CAD build for the part. Positions are in the model's coordinates, mm. A direction names the side the tool comes from. Coordinates: 2 decimals unless noted, no trailing zeros. Order: outer loops, then holes, each group sorted by start corner. A loop starts at its lowest first (then second) coordinate and runs counter-clockwise, first axis right, second up.
from build123d import *

# Parameters (mm, degrees)
PAD_DEPTH     = 2.5
SKETCH002_W   = 6.25
SKETCH002_H   = 30
SKETCH002_W_2 = 10
SKETCH002_H_2 = 35
POCKET_DEPTH  = 1.5


with BuildPart() as part:
    # Sketch → Pad (new body)
    with BuildSketch(Plane.XY):
        Polygon((-10, 14.125), (5, 14.125), (12.25, 7.5), (102.25, 7.5), (102.25, -7.5), (12.25, -7.5), (5, -14.125), (-10, -14.125), (-10, -9.125), (0, -9.125), (0, 9.125), (-10, 9.125), align=None)
    extrude(amount=PAD_DEPTH)

    # Sketch002 → Pocket (cut)
    with BuildSketch(Plane.XY.offset(2.5)):
        with Locations((94.125, 0)):
            Rectangle(SKETCH002_W, SKETCH002_H)
        with Locations((-7, 0)):
            Rectangle(SKETCH002_W_2, SKETCH002_H_2)
    extrude(amount=-POCKET_DEPTH, mode=Mode.SUBTRACT)


solid = part.part
1) Which spindle directions (+Z, -Z, +X, -X, +Y, -Y) get a long thin tool onto all of the face, cutting with end or side? Do faces 4 (the flat face through (57, 7.5, 1)), 5 (the flat face through (58, -7.5, 1)), 6 (the flat face through (-3.8, 9.125, 0.7)), 7 (the flat face through (-6, -12, 1)). Say none if no direction does.
2) Slice it at B-B (y = 4.75). List the corners of the cut face in (x, z), plus the area to 3 significant figures.
3) Drill centre lines: probe 1 along X at (y, z) = (0, 2); probe 2 along Y at (x, z) = (76, 1.2); probe 3 along X at (y, z) = (-1.5, 0.15). Where is each one in solid material? Low to high.
4) Slice it at A-A (z = 1.75). List the corners of the cut face in (x, y) (3 decimals), plus the area to 3 significant figures.
5) Slice it at C-C (x = 79.5). List the corners of the cut face in (y, z).
6) Slice it at D-D (y = -10.5). List the corners of the cut face in (x, z), plus the area to 3 significant figures.
7) Two-plate mould, pull along Y, no slides. Class faces 1 (the flat face through (-6, 12, 1)), 2 (the flat face through (-1, -14.125, 1)), 3 (the flat face through (0, 0, 1)): released by +Y, released by -Y, zero draft, split by the parting line, or undercut.
8) Pin check, flat tips, straight feed: P1, Ø1.5, axis at x = 26, z = 1.5, coming from the -Y side; P2, Ø5.5, axis at x = -6, y = -10.5, coming from the +Z side; P3, Ø0.8, axis at y = -2, z = 2, coming from the -X side. Stop position of each tip, or through.
Worked out:
1. face 4: +Z, -Z, +X, +Y
1. face 5: +Z, -Z, +X, -Y
1. face 6: +Z, -Z, -X
1. face 7: +Z, -X, +Y, -Y
2. outline: (0, 0) - (102.25, 0) - (102.25, 2.5) - (97.25, 2.5) - (97.25, 1) - (91, 1) - (91, 2.5) - (0, 2.5) - close
2. area: 246 mm2
3. probe 1: x = 0 to 91, 97.25 to 102.25
3. probe 2: y = -7.5 to 7.5
3. probe 3: x = 0 to 102.25
4. outline: (-2, -14.125) - (5, -14.125) - (12.25, -7.5) - (91, -7.5) - (91, 7.5) - (12.25, 7.5) - (5, 14.125) - (-2, 14.125) - (-2, 9.125) - (0, 9.125) - (0, -9.125) - (-2, -9.125) - close; (97.25, -7.5) - (102.25, -7.5) - (102.25, 7.5) - (97.25, 7.5) - close
4. area: 1,570 mm2
5. outline: (-7.5, 0) - (7.5, 0) - (7.5, 2.5) - (-7.5, 2.5) - close
6. outline: (-10, 0) - (8.97, 0) - (8.97, 2.5) - (-2, 2.5) - (-2, 1) - (-10, 1) - close
6. area: 35.4 mm2
7. face 1: zero draft
7. face 2: released by -Y
7. face 3: undercut
8. P1: stops at y = -7.5
8. P2: stops at z = 1
8. P3: stops at x = 0
